Answer from the drawing. Dimensions are ordinates in mm from the lowest x, y and z of the part. A direction names the side the tool comes from. Coordinates: 2 decimals unless noted, no trailing zeros. Write each loop counter-clockwise with the first axis right and the second up, starting at its lowest first coordinate (ties: lowest second). Pieces come first, ordered by that corner, then holes. Notation, with made-up numbers: (-35.75, -39) -> (20.25, -39) arc R19 ccw to (20.25, -29) -> close; hole circle Ø7 at (42.25, 89.5). An arc over 180 degrees is marked (long way). Return JSON: item names as keys, results as strings.
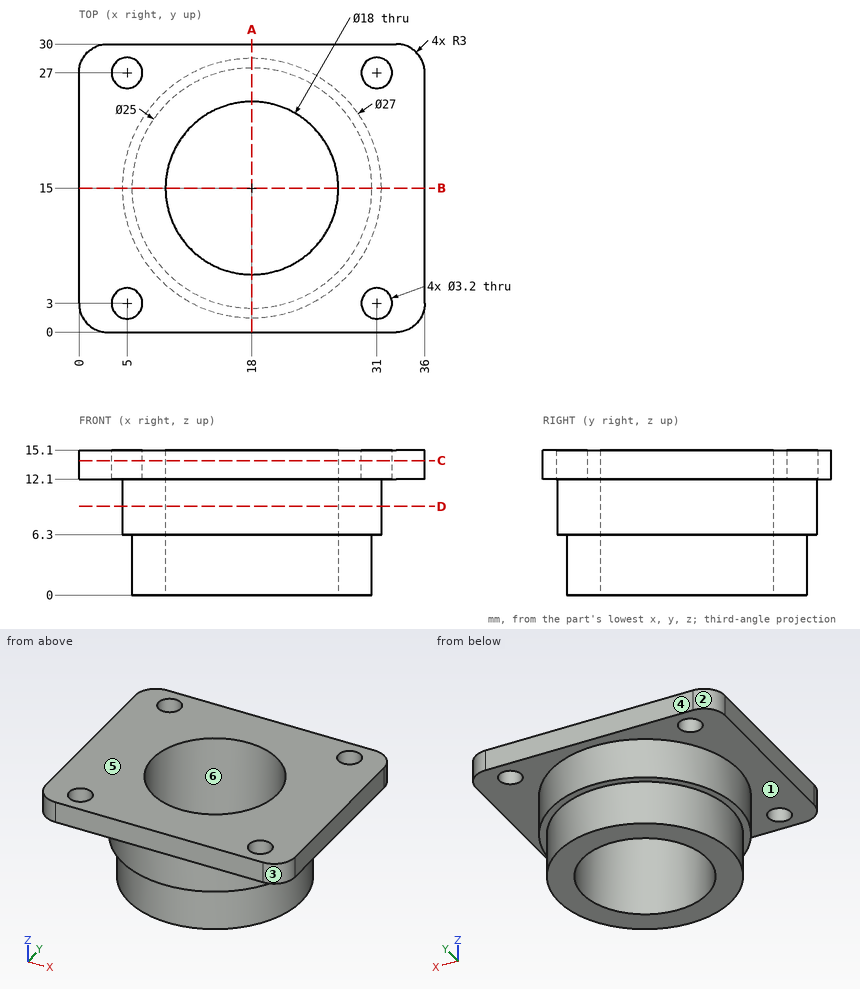
1. A tool of negligible diameter and unlimited length cuts with its end or side. For the marked faces 1 and 2, from which of +Z, -Z, +X, -X, +Y, -Y can it reach the whole face along a straight path? Write none if from no direction.
Taken from the geometry:
{"face 1": "-Z", "face 2": "+Z, -Z, -X, +Y"}
2. For a pull along Y with two mould halves and no side action, classify the marked faces 3, 4, 5 and 6 as +Y half, -Y half, draft (parallel to the pull), parting line (faces both ways), or undercut.
Taken from the geometry:
{"face 3": "-Y half", "face 4": "+Y half", "face 5": "draft", "face 6": "undercut"}
3. Consider L1, parallel to Y at x = 31, z = 12.9; L2, parallel to Y at x = 18, z = 8.75; L3, parallel to Z at x = 2, y = 18.25. Determine where each line is inside the solid, lowest interval first.
Taken from the geometry:
{"L1": "y = 0 to 1.4, 4.6 to 25.4, 28.6 to 30", "L2": "y = 1.5 to 6, 24 to 28.5", "L3": "z = 12.1 to 15.1"}
4. The part is cut by section C-C (z = 14). Determine the outline of the cut face in (x, y).
Taken from the geometry:
{"outline": "(0, 3) arc R3 ccw to (3, 0) -> (33, 0) arc R3 ccw to (36, 3) -> (36, 27) arc R3 ccw to (33, 30) -> (3, 30) arc R3 ccw to (0, 27) -> close; hole circle Ø3.2 at (5, 3); hole circle Ø3.2 at (5, 27); hole circle Ø18 at (18, 15); hole circle Ø3.2 at (31, 3); hole circle Ø3.2 at (31, 27)"}
5. The part is cut by section D-D (z = 9.25). Determine the outline of the cut face in (x, y), then the cut area to 3 significant figures.
Taken from the geometry:
{"outline": "circle Ø27 at (18, 15); hole circle Ø18 at (18, 15)", "area": "318 mm2"}
6. The part is cut by section B-B (y = 15). Determine the outline of the cut face in (x, z), then the cut area to 3 significant figures.
Taken from the geometry:
{"outline": "(0, 12.1) -> (4.5, 12.1) -> (4.5, 6.3) -> (5.5, 6.3) -> (5.5, 0) -> (9, 0) -> (9, 15.1) -> (0, 15.1) -> close; (27, 0) -> (30.5, 0) -> (30.5, 6.3) -> (31.5, 6.3) -> (31.5, 12.1) -> (36, 12.1) -> (36, 15.1) -> (27, 15.1) -> close", "area": "150 mm2"}
7. Flat-ended cylindrical pins translate along their axes: pin 1 Ø1 at (y, z) = (24, 8) entering from +X; pin 2 Ø1.5 at (y, z) = (19.5, 7.5) entering from -X; pin 3 Ø6 at (y, z) = (8, 6.5) entering from -X. Find the tip coordinate at first contact, or state that the pin passes through.
Taken from the geometry:
{"pin 1": "stops at x = 28.49", "pin 2": "stops at x = 5.03", "pin 3": "stops at x = 5.11"}
8. The part is cut by section A-A (x = 18). Determine the outline of the cut face in (y, z).
Taken from the geometry:
{"outline": "(0, 12.1) -> (1.5, 12.1) -> (1.5, 6.3) -> (2.5, 6.3) -> (2.5, 0) -> (6, 0) -> (6, 15.1) -> (0, 15.1) -> close; (24, 0) -> (27.5, 0) -> (27.5, 6.3) -> (28.5, 6.3) -> (28.5, 12.1) -> (30, 12.1) -> (30, 15.1) -> (24, 15.1) -> close"}
